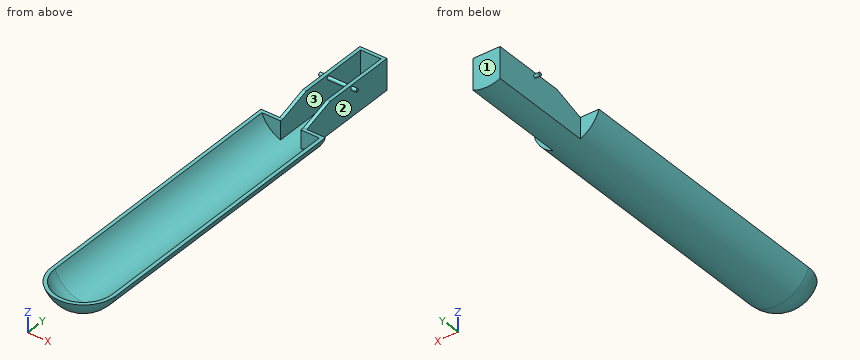
```python
from build123d import *

# Parameters (mm, degrees)
F1_ANGLE_BACK = 90
F1_ANGLE      = 180
F3_DEPTH      = 1016
F5_DEPTH      = 12.7
F7_DEPTH      = 381
F9_DEPTH      = 12.7
F11_DEPTH     = 127
F12_R         = 6.35
F13_DEPTH     = 69.85


with BuildPart() as f1:
    # F0 (on Right) → F1 (revolve)
    with BuildSketch(Plane.YZ, mode=Mode.PRIVATE) as f1_sk:
        with BuildLine():
            Line((-622.3, 0), (-635, 0))
            ThreePointArc((-635, 0), (-597.8025612107, -89.8025612107), (-508, -127))
            Line((-508, -127), (-508, -114.3))
            ThreePointArc((-508, -114.3), (-588.8223050896, -80.8223050896), (-622.3, 0))
        make_face()
    revolve(f1_sk.sketch.rotate(Axis((0, -628.65, 0), (0, -1, 0)), -F1_ANGLE_BACK), axis=Axis((0, -628.65, 0), (0, -1, 0)), revolution_arc=F1_ANGLE)

    # F2 (on face) → F3 (join)
    with BuildSketch(Plane(origin=(0, -508, 0), x_dir=(-1, 0, 0), z_dir=(0, 1, 0))):
        with BuildLine():
            Line((-114.3, 0), (-127, 0))
            ThreePointArc((-127, 0), (0, -127), (127, 0))
            Line((127, 0), (114.3, 0))
            ThreePointArc((114.3, 0), (0, -114.3), (-114.3, 0))
        make_face()
    extrude(amount=F3_DEPTH)

    # F4 (on face) → F5 (join)
    with BuildSketch(Plane(origin=(0, 508, 0), x_dir=(-1, 0, 0), z_dir=(0, 1, 0))):
        with BuildLine():
            Line((-38.1, 0), (-127, 0))
            ThreePointArc((-127, 0), (0, -127), (127, 0))
            Line((127, 0), (38.1, 0))
            Line((38.1, 0), (38.1, -107.7630734528))
            ThreePointArc((38.1, -107.7630734528), (0, -114.3), (-38.1, -107.7630734528))
            Line((-38.1, -107.7630734528), (-38.1, 0))
        make_face()
    extrude(amount=F5_DEPTH)

    # F6 (on face) → F7 (join)
    with BuildSketch(Plane(origin=(0, 520.7, 0), x_dir=(-1, 0, 0), z_dir=(0, 1, 0))):
        with BuildLine():
            Line((-38.1, 0), (-50.8, 0))
            Line((-50.8, 0), (-50.8, -116.3974226519))
            ThreePointArc((-50.8, -116.3974226519), (0, -127), (50.8, -116.3974226519))
            Line((50.8, -116.3974226519), (50.8, 0))
            Line((50.8, 0), (38.1, 0))
            Line((38.1, 0), (38.1, -107.7630734528))
            ThreePointArc((38.1, -107.7630734528), (0, -114.3), (-38.1, -107.7630734528))
            Line((-38.1, -107.7630734528), (-38.1, 0))
        make_face()
    extrude(amount=F7_DEPTH)

    # F8 (on face) → F9 (join)
    with BuildSketch(Plane(origin=(0, 901.7, 0), x_dir=(-1, 0, 0), z_dir=(0, 1, 0))):
        with BuildLine():
            Line((-50.8, 0), (-50.8, -116.3974226519))
            ThreePointArc((-50.8, -116.3974226519), (0, -127), (50.8, -116.3974226519))
            Line((50.8, -116.3974226519), (50.8, 0))
            Line((50.8, 0), (-50.8, 0))
        make_face()
    extrude(amount=F9_DEPTH)

    # F10 (on Right) → F11 (cut, symmetric)
    with BuildSketch(Plane.YZ):
        with BuildLine():
            Line((635, 0), (-635, 0))
            ThreePointArc((-635, 0), (-633.5290511787, -19.2732278089), (-629.15027858, -38.1))
            Line((-629.15027858, -38.1), (520.7, -38.1))
            Line((520.7, -38.1), (635, 0))
        make_face()
    extrude(amount=F11_DEPTH, both=True, mode=Mode.SUBTRACT)

    # F12 (on Right) → F13 (join, symmetric)
    with BuildSketch(Plane.YZ):
        with Locations((742.95, -12.7)):
            Circle(F12_R)
    extrude(amount=F13_DEPTH, both=True)


solid = f1.part
```
Here's how the part is built. I have some questions about the finished solid (model axes, mm). Face numbers are marked on the shaded views. Coordinates: 2 decimals unless noted, no trailing zeros. Write each loop counter-clockwise with the first axis right and the second up, starting at its lowest first coordinate (ties: lowest second). Pieces come first, ordered by that corner, then holes. Notation, with made-up numbers: (18.25, 56) -> (23.25, 56) arc R29 cw to (23.25, 84) -> close; hole circle Ø6 at (3, -14). An arc over 180 degrees is marked (long way). Use a Markdown table: item, result. Add a question column.
(1) If we section it at D-D, the plane x = -82.5: Write out the boundary of the cut face in (y, z).
(2) If we section it at C-C, the plane y = 800: Write out the boundary of the cut face in (x, z), and give its area (3 significant figures).
(3) Please list where these lines run through material, in increasing order: line 1 (X direction, y = 530, z = -42); line 2 (X direction, y = -478, z = -89.5); line 3 (Y direction, x = 36, z = -17).
(4) I'm going to push flat-ended pins straight in: P1, Ø2, axis at y = 757, z = -20.5, coming from the +X side; P2, Ø8, axis at y = -112, z = -72.5, coming from the -X side; P3, Ø1.5, axis at y = 179.5, z = -56.5, coming from the +X side. Where does each tip first touch, or does it pass through?
(5) If we section it at A-A, the plane x = -25: Write out the boundary of the cut face in (y, z), and give its area (3 significant figures).
(6) If we section it at B-B, the plane z = -62: Write out the boundary of the cut face in (x, y), and give its area (3 significant figures).
(7) We'd pull the mould along Y, two halves only. Please class the marked faces 1, 2 and 3: +Y half, -Y half, draft (parallel to the pull), parting line (faces both ways), or undercut.
Outcome:
| question | item | result |
|---|---|---|
| 1 | outline | (-596.72, -38.1) arc R96.55 ccw to (-508, -96.55) -> (520.7, -96.55) -> (520.7, -38.1) -> (508, -38.1) -> (508, -79.11) -> (-508, -79.11) arc R79.11 cw to (-577.33, -38.1) -> close |
| 2 | outline | (-50.8, -116.4) arc R127 ccw to (50.8, -116.4) -> (50.8, 0) -> (38.1, 0) -> (38.1, -107.76) arc R114.3 cw to (-38.1, -107.76) -> (-38.1, 0) -> (-50.8, 0) -> close |
| 2 | area | 4,000 mm^2 |
| 3 | line 1 | x = -50.8 to -38.1, 38.1 to 50.8 |
| 3 | line 2 | x = -90.1 to -71.09, 71.09 to 90.1 |
| 3 | line 3 | y = 738.28 to 747.62, 901.7 to 914.4 |
| 4 | P1 | stops at x = 50.8 |
| 4 | P2 | stops at x = -106.94 |
| 4 | P3 | stops at x = 114.11 |
| 5 | outline | (-626.54, -38.1) arc R124.52 ccw to (-508, -124.52) -> (914.4, -124.52) -> (914.4, 0) -> (901.7, 0) -> (901.7, -111.53) -> (-508, -111.53) arc R111.53 cw to (-612.82, -38.1) -> close; circle Ø12.7 at (742.95, -12.7) |
| 5 | area | 21,900 mm^2 |
| 6 | outline | (-110.84, -508) arc R110.84 ccw to (110.84, -508) -> (110.84, 520.7) -> (50.8, 520.7) -> (50.8, 914.4) -> (-50.8, 914.4) -> (-50.8, 520.7) -> (-110.84, 520.7) -> close; hole (-96.02, -508) arc R96.02 ccw to (96.02, -508) -> (96.02, 508) -> (38.1, 508) -> (38.1, 901.7) -> (-38.1, 901.7) -> (-38.1, 508) -> (-96.02, 508) -> close |
| 6 | area | 47,700 mm^2 |
| 7 | face 1 | +Y half |
| 7 | face 2 | draft |
| 7 | face 3 | undercut |
